from build123d import *

# Parameters (mm, degrees)
SKETCH1_W           = 5
SKETCH1_H           = 1.5
BOSS_EXTRUDE1_DEPTH = 2


with BuildPart() as part:
    # Sketch1 → Revolve1 (revolve)
    with BuildSketch(Plane.XY):
        with Locations((0, 0.75)):
            Rectangle(SKETCH1_W, SKETCH1_H)
    revolve(axis=Axis((-16.166606446, 0, 0), (1, 0, 0)))

    # Sketch2 → Boss-Extrude1 (add)
    with BuildSketch(Plane(origin=(2.5, 0, 0), x_dir=(0, 0, -1), z_dir=(1, 0, 0))):
        Polygon((1.58771324, 2.75), (-1.58771324, 2.75), (-3.175426481, 0), (-1.58771324, -2.75), (1.58771324, -2.75), (3.175426481, 0), align=None)
    extrude(amount=BOSS_EXTRUDE1_DEPTH)


solid = part.part
Design review of the part built by this model. Coordinates are the model's own, in mm. A direction names the side the tool comes from. Give positions to 0.01 mm unless a question says otherwise; leave off trailing zeros. Order: outer loops, then holes, each group sorted by start corner. A loop starts at its lowest first (then second) coordinate and runs counter-clockwise, first axis right, second up. Notation, with made-up numbers: (17, 29) - (75, 29) arc R27 cw to (75, 65) - close; hole circle Ø2 at (4, 74). An arc over 180 degrees is marked (long way). Write item = value, one per line. Start each with the question number.
Q1. To check wall thickness, follow L1, parallel to X at y = 2.3, z = -0.75; L2, parallel to Y at x = 1.75, z = 0.5; L3, parallel to Z at x = -1.25, y = -0.65. State the ranges of each line that lie inside material, in increasing order. Write a range as from..to.
Q2. We need section B-B on x = 4. State the section outline as (y, z) points, plus the area to 3 significant figures.
Q3. We need section A-A on z = -0.25. State the section outline as (x, y) points, plus the area to 3 significant figures.
Q4. Tool access review of faces 1 (the face through (3.486, -1.394, -2.37)), 2 (the face through (2.5, 1.3, -1.4)): name each direction out of +Z, -Z, +X, -X, +Y, -Y from which nothing blocks a thin tool from reaching the whole face with its end or side.
Q5. Clearance check with a flat-ended pin moving along its axis: pin 1 Ø1.5 at (x, z) = (3.5, -2.5) entering from -Y. State where the tip first meets the part, or that it passes through.
Q6. We need section C-C on y = 1.3. State the section outline as (x, z) points.
Q7. We need section D-D on x = 1.25. State the section outline as (y, z) points.
Working result:
q1.L1 = 2.5..4.5
q1.L2 = -1.41..1.41
q1.L3 = -1.35..1.35
q2.outline = (-2.75, -1.59) - (0, -3.18) - (2.75, -1.59) - (2.75, 1.59) - (0, 3.18) - (-2.75, 1.59) - close
q2.area = 26.2 mm²
q3.outline = (-2.5, -1.48) - (2.5, -1.48) - (2.5, -2.75) - (4.5, -2.75) - (4.5, 2.75) - (2.5, 2.75) - (2.5, 1.48) - (-2.5, 1.48) - close
q3.area = 25.8 mm²
q4.face_1 = -Z, +X, -X, -Y
q4.face_2 = -X
q5.pin_1 = -2.47
q6.outline = (-2.5, -0.75) - (2.5, -0.75) - (2.5, -2.42) - (4.5, -2.42) - (4.5, 2.42) - (2.5, 2.42) - (2.5, 0.75) - (-2.5, 0.75) - close
q7.outline = circle Ø3 at (0, 0)
